```python
from build123d import *

# Parameters (mm, degrees)
SKETCH_3_W          = 20
SKETCH_3_H          = 20
SKETCH_3_R          = 4
EXTRUDE_2_DEPTH     = 6
SKETCH_4_R          = 1
CUT_EXTRUDE_1_DEPTH = 6
HOLE_WIZARD_M3_1_D  = 2.5
HOLE_WIZARD_M3_2_D  = 2.5
FILLET_1_R          = 2
HOLE_WIZARD_M3_3_D  = 2.5


with BuildPart() as part:
    # 草图3 → 凸台-拉伸2 (new body)
    with BuildSketch(Plane(origin=(0, 0, 0), x_dir=(0, 0, -1), z_dir=(1, 0, 0))):
        Rectangle(SKETCH_3_W, SKETCH_3_H)
        Circle(SKETCH_3_R, mode=Mode.SUBTRACT)
    extrude(amount=EXTRUDE_2_DEPTH)

    # 草图4 → 切除-拉伸1 (cut)
    with BuildSketch(Plane(origin=(6, 0, 0), x_dir=(0, 0, -1), z_dir=(1, 0, 0))):
        with Locations((-7, 7)):
            Circle(SKETCH_4_R)
        with Locations((7, 7)):
            Circle(SKETCH_4_R)
        with Locations((-7, -7)):
            Circle(SKETCH_4_R)
        with Locations((7, -7)):
            Circle(SKETCH_4_R)
    extrude(amount=-CUT_EXTRUDE_1_DEPTH, mode=Mode.SUBTRACT)

    # M3 螺纹孔1 (through all)
    with Locations(Plane(origin=(0, 10, 0), x_dir=(1, 0, 0), z_dir=(0, 1, 0))):
        with Locations((3, 0)):
            Hole(HOLE_WIZARD_M3_1_D / 2)

    # M3 螺纹孔2 (through all)
    with Locations(Plane(origin=(0, 0, -10), x_dir=(-1, 0, 0), z_dir=(0, 0, -1))):
        with Locations((-3, 0)):
            Hole(HOLE_WIZARD_M3_2_D / 2)

    # 圆角1
    fillet_1_edges = [part.edges().sort_by_distance(p)[0] for p in [
        (3, 10, 10),
        (3, 10, -10),
        (3, -10, -10),
        (3, -10, 10),
    ]]
    fillet(fillet_1_edges, radius=FILLET_1_R)

    # M3 螺纹孔3 (through all)
    with Locations(Plane.ZY):
        with Locations((-7, 7), (7, 7), (-7, -7), (7, -7)):
            Hole(HOLE_WIZARD_M3_3_D / 2)


solid = part.part
```
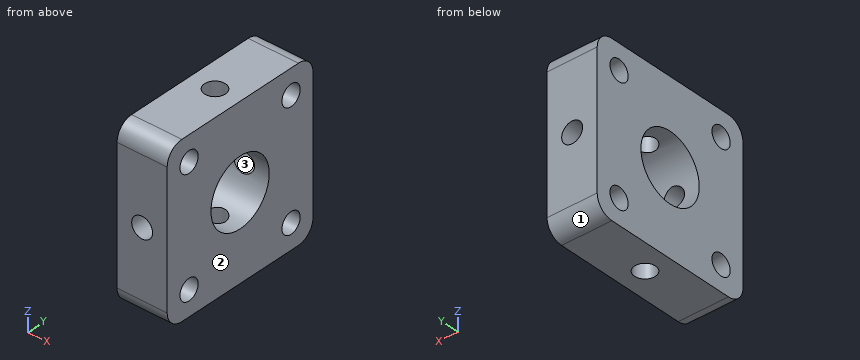
Build history of the part. All positions in model axes, mm. Face numbers are marked on the shaded views. Give positions to 0.01 mm unless a question says otherwise; leave off trailing zeros. Loops run counter-clockwise (first coordinate to the right, second up) from the corner with the lowest first, then second, coordinate; pieces in that order, holes last.
Item 1: Pull direction X, two halves, no side cores. Call the marked faces 1, 2 and 3: released by +X, released by -X, zero draft, split by the parting line, or undercut.
Answers follow:
face 1: zero draft
face 2: released by +X
face 3: undercut
Item 2: Flat gauge pins, fed straight in: pin 1 (1.5 mm diameter, centred on x = 3, z = 0, fed in from -Y) (3 decimals); pin 2 (3 mm diameter, centred on x = 3, y = 0, fed in from +Z). Where does each tip first touch, or does it go through?
Answers follow:
pin 1: passes through
pin 2: stops at z = 10
Item 3: Slice it at D-D, the plane y = 0. List the corners of the cut face in (x, z).
Answers follow:
outline: (0, -10) - (1.75, -10) - (1.75, -4) - (0, -4) - close; (0, 4) - (1.75, 4) - (1.75, 10) - (0, 10) - close; (4.25, -10) - (6, -10) - (6, -4) - (4.25, -4) - close; (4.25, 4) - (6, 4) - (6, 10) - (4.25, 10) - close
Item 4: Slice it at A-A, the plane y = -7. List the corners of the cut face in (x, z).
Answers follow:
outline: (0, -10) - (6, -10) - (6, -8.25) - (0, -8.25) - close; (0, -5.75) - (6, -5.75) - (6, 5.75) - (0, 5.75) - close; (0, 8.25) - (6, 8.25) - (6, 10) - (0, 10) - close; hole circle Ø2.5 at (3, 0)
Item 5: Drill centre lines: line 1 (Z direction, x = 3, y = -4.5); line 2 (X direction, y = 0, z = 6.25); line 3 (Y direction, x = 5.5, z = 1.25). Where is each one in solid material? Low to high.
Answers follow:
line 1: z = -10 to -1.25, 1.25 to 10
line 2: x = 0 to 1.75, 4.25 to 6
line 3: y = -10 to -3.8, 3.8 to 10
Item 6: Slice it at C-C, the plane x = 3. List the corners of the cut face in (y, z).
Answers follow:
outline: (-10, -8) arc R2 ccw to (-8, -10) - (-1.25, -10) - (-1.25, -3.8) arc R4 cw to (-3.8, -1.25) - (-10, -1.25) - close; (-10, 1.25) - (-3.8, 1.25) arc R4 cw to (-1.25, 3.8) - (-1.25, 10) - (-8, 10) arc R2 ccw to (-10, 8) - close; (1.25, -10) - (8, -10) arc R2 ccw to (10, -8) - (10, -1.25) - (3.8, -1.25) arc R4 cw to (1.25, -3.8) - close; (1.25, 3.8) arc R4 cw to (3.8, 1.25) - (10, 1.25) - (10, 8) arc R2 ccw to (8, 10) - (1.25, 10) - close; hole circle Ø2.5 at (-7, -7); hole circle Ø2.5 at (-7, 7); hole circle Ø2.5 at (7, -7); hole circle Ø2.5 at (7, 7)
